```python
from build123d import *

# Parameters (mm, degrees)
F0_R     = 2.75
F0_R_2   = 1.5
F1_DEPTH = 3.15
F2_DEPTH = 10
F4_DEPTH = 3


with BuildPart() as f1:
    # F0 (on Top) → F1 (new body)
    with BuildSketch(Plane.XY):
        Circle(F0_R)
        Circle(F0_R_2, mode=Mode.SUBTRACT)
    extrude(amount=F1_DEPTH)

    # F0 (on Top) → F2 (join)
    with BuildSketch(Plane.XY):
        Circle(F0_R_2)
    extrude(amount=F2_DEPTH)

    # F3 (on face) → F4 (cut)
    with BuildSketch(Plane(origin=(0, 0, 0), x_dir=(1, 0, 0), z_dir=(0, 0, -1))):
        Polygon((1.349507, 1.524745), (-0.598857, 1.958133), (-1.948365, 0.487494), (-1.349507, -1.416534), (0.598857, -1.849922), (1.948365, -0.379282), align=None)
    extrude(amount=-F4_DEPTH, mode=Mode.SUBTRACT)


solid = f1.part
```
Work out the finished part from the listing and answer in its coordinate system (mm). A direction names the side the tool comes from. Give positions to 0.01 mm unless a question says otherwise; leave off trailing zeros. Order: outer loops, then holes, each group sorted by start corner. A loop starts at its lowest first (then second) coordinate and runs counter-clockwise, first axis right, second up.
1. Section C-C, the plane y = 0.85 is taken. Determine the outline of the cut face in (x, z), and give its area (3 significant figures).
Result sheet:
outline: (-2.62, 0) - (-1.53, 0) - (-1.53, 3) - (1.52, 3) - (1.52, 0) - (2.62, 0) - (2.62, 3.15) - (1.24, 3.15) - (1.24, 10) - (-1.24, 10) - (-1.24, 3.15) - (-2.62, 3.15) - close
area: 24.3 mm2
2. Straight lines are drawn through the part: L1, parallel to Z at x = -2.3, y = 0.25; L2, parallel to X at y = 0.1, z = 2.25; L3, parallel to Z at x = 0.1, y = -0.75. For each, find the intervals that lie inside material, in ascending order.
Result sheet:
L1: z = 0 to 3.15
L2: x = -2.75 to -1.76, 1.86 to 2.75
L3: z = 3 to 10
3. For faces 1 (the flat face through (-0.39, 1.63, 1.48)), 2 (the cylindrical face through (-0.596, -2.685, 1.553)), 3 (the flat face through (2, 0, 3.15)), determine the directions among +Z, -Z, +X, -X, +Y, -Y from which every point of the face is accessible in a straight line to the end or side of a thin tool.
Result sheet:
face 1: -Z
face 2: +Z, -Z
face 3: +Z
4. Section B-B, the plane x = -0.05 is taken. Determine the outline of the cut face in (y, z).
Result sheet:
outline: (-2.75, 0) - (-1.84, 0) - (-1.84, 3) - (1.71, 3) - (1.71, 0) - (2.75, 0) - (2.75, 3.15) - (1.5, 3.15) - (1.5, 10) - (-1.5, 10) - (-1.5, 3.15) - (-2.75, 3.15) - close
5. The mould has two halves that part along Y. Classify faces 4 (the flat face through (-1.653, 0.451, 1.479)), 5 (the flat face through (-1.264, -1.233, 1.479)), 6 (the flat face through (0, 0, 10)), 7 (the cylindrical face through (-1.5, 0.07, 6.53)): released by +Y, released by -Y, zero draft, split by the parting line, or undercut.
Result sheet:
face 4: undercut
face 5: undercut
face 6: zero draft
face 7: split by the parting line
6. This flat-tipped pin is pushed along its axis until it touches: P1, Ø1.5, axis at y = -0.5, z = 9, coming from the +X side. Where does it stop, or does it pass through?
Result sheet:
P1: stops at x = 1.5
7. Section A-A, the plane z = 2 is taken. Determine the outline of the cut face in (x, y).
Result sheet:
outline: circle Ø5.5 at (0, 0); hole (-1.95, -0.49) - (-0.6, -1.96) - (1.35, -1.52) - (1.95, 0.38) - (0.6, 1.85) - (-1.35, 1.42) - close
8. Section D-D, the plane z = 8.75 is taken. Determine the outline of the cut face in (x, y).
Result sheet:
outline: circle Ø3 at (0, 0)
